Here's the drawing with two shaded views (mm, measured from the low corner). I have some questions. A direction names the side the tool comes from. Round coordinates to 2 decimals unless told otherwise and drop trailing zeros. Loops run counter-clockwise (first coordinate to the right, second up) from the corner with the lowest first, then second, coordinate; pieces in that order, holes last. Notation, with made-up numbers: (76.25, 57.5) - (126.25, 57.5) arc R31 ccw to (126.25, 87.5) - close; hole circle Ø1 at (30.5, 60.5). An arc over 180 degrees is marked (long way). Use one line per item in the form item = value.
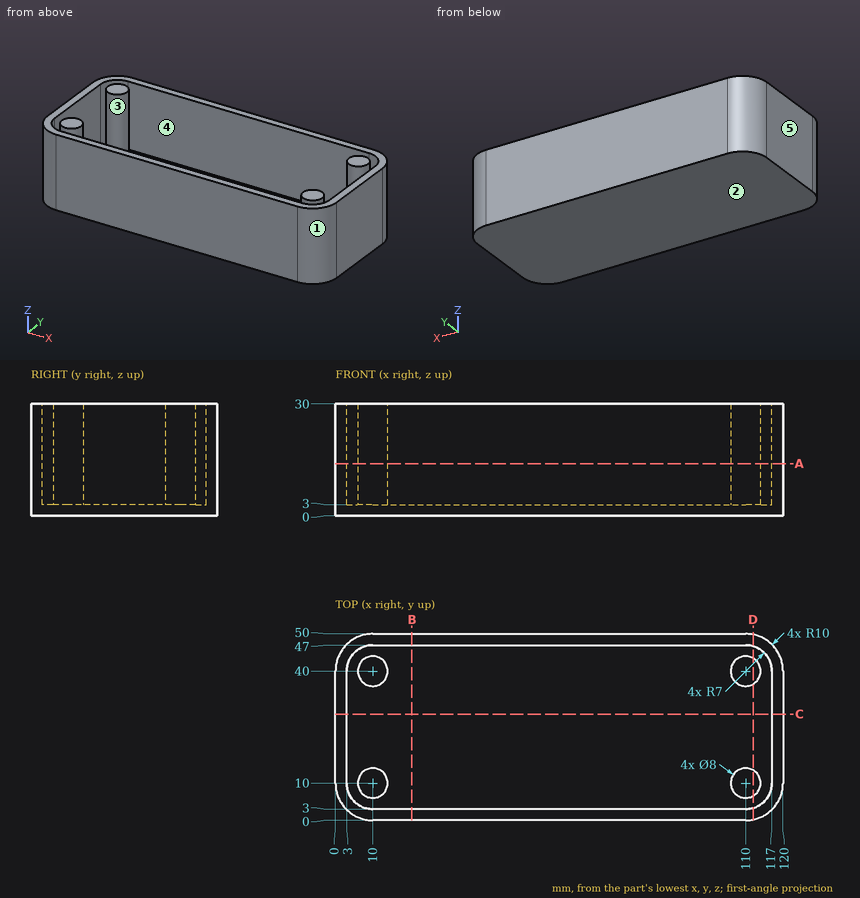
1. For P1, Ø5, axis at x = 79, y = 22.5, coming from the +Z side, with a flat end and sliding along its axis, tell me the tip position at first contact or that it passes through.
Solution:
P1 = 3
2. We'd pull the mould along X, two halves only. Please class the marked faces 1, 2 and 3: +X half, -X half, draft (parallel to the pull), parting line (faces both ways), or undercut.
Solution:
face_1 = +X half
face_2 = draft
face_3 = undercut
3. Please list where these lines run through material, in increasing order: line 1 along Y through (x, z) = (41.5, 6); line 2 along Y through (x, z) = (9.5, 16); line 3 along X through (y, z) = (43.5, 22.75).
Solution:
line_1 = 0 to 3, 47 to 50
line_2 = 0.01 to 3.02, 6.03 to 13.97, 36.03 to 43.97, 46.98 to 49.99
line_3 = 0.63 to 3.94, 8.06 to 11.94, 108.06 to 111.94, 116.06 to 119.37
4. If we section it at C-C, the plane y = 28.5: Write out the boundary of the cut face in (x, z).
Solution:
outline = (0, 0) - (120, 0) - (120, 30) - (117, 30) - (117, 3) - (3, 3) - (3, 30) - (0, 30) - close
5. If we section it at B-B, the plane x = 20.5: Write out the boundary of the cut face in (y, z).
Solution:
outline = (0, 0) - (50, 0) - (50, 30) - (47, 30) - (47, 3) - (3, 3) - (3, 30) - (0, 30) - close
6. If we section it at D-D, the plane x = 112: Write out the boundary of the cut face in (y, z), plus the area to 3 significant figures.
Solution:
outline = (0.2, 0) - (49.8, 0) - (49.8, 30) - (46.71, 30) - (46.71, 3) - (43.46, 3) - (43.46, 30) - (36.54, 30) - (36.54, 3) - (13.46, 3) - (13.46, 30) - (6.54, 30) - (6.54, 3) - (3.29, 3) - (3.29, 30) - (0.2, 30) - close
area = 690 mm^2
7. If we section it at A-A, the plane z = 14: Write out the boundary of the cut face in (x, y).
Solution:
outline = (0, 10) arc R10 ccw to (10, 0) - (110, 0) arc R10 ccw to (120, 10) - (120, 40) arc R10 ccw to (110, 50) - (10, 50) arc R10 ccw to (0, 40) - close; circle Ø8 at (10, 10); circle Ø8 at (10, 40); circle Ø8 at (110, 10); circle Ø8 at (110, 40); hole (3, 10) arc R7 ccw to (10, 3) - (110, 3) arc R7 ccw to (117, 10) - (117, 40) arc R7 ccw to (110, 47) - (10, 47) arc R7 ccw to (3, 40) - close
8. On a 3-axis mill with a long thin cutter (end or side, diameter ignored), from which of +Z, -Z, +X, -X, +Y, -Y can I reach the whole of each face in a straight line? I mean the marked faces 4 and 5. Say none if no direction works.
Solution:
face_4 = +Z
face_5 = +Z, -Z, -X, +Y, -Y
